Can you work these out from the model? Positions are in its coordinate system, mm. A direction names the side the tool comes from. Coordinates: 2 decimals unless noted, no trailing zeros. Order: outer loops, then holes, each group sorted by start corner. A loop starts at its lowest first (then second) coordinate and runs counter-clockwise, first axis right, second up.
Autodesk Inventor part; units mm, degrees
ref_plane "Work Plane1" through (220.5144, 586.5816, 98.3522) normal (0, 0, 1) x (1, 0, 0)
ref_plane "YZ Plane" through (0, 0, 0) normal (1, 0, 0) x (0, 1, 0)
ref_plane "XZ Plane" through (0, 0, 0) normal (0, 1, 0) x (-1, 0, 0)
ref_plane "Work Plane1" through (220.5144, 586.5816, 98.3522) normal (0, 0, 1) x (1, 0, 0)
sketch "Sketch1" plane through (220.5144, 586.5816, 98.3522) normal (0, 0, 1) x (1, 0, 0)
  line L0 (12.7, 622.3) -> (215.9, 622.3)
  line L1 (12.7, 317.5) -> (215.9, 317.5)
  line L2 (241.3, 317.5) -> (241.3, 596.9)
  line L3 (-12.7, 596.9) -> (-12.7, 317.5)
  line L4 (215.9, 596.9) -> (12.7, 596.9)
  line L5 (215.9, 596.9) -> (215.9, 317.5)
  line L6 (12.7, 317.5) -> (12.7, 596.9)
  line L7 (212.725, 593.725) -> (15.875, 593.725)
  line L8 (15.875, 593.725) -> (15.875, 320.675)
  line L9 (15.875, 320.675) -> (212.725, 320.675)
  line L10 (212.725, 320.675) -> (212.725, 593.725)
  point P0 (-220.5144, -586.5816)
extrude "Extrusion1" add sketch "Sketch1" along normal blind 127 and the other way blind 25.4 contours L10 L9 L8 L7
shell "Shell1" thickness 12.7 removed faces 1 at (302.006, 1089.2899, 225.3522)
sketch "Sketch2" plane through (433.2394, 907.2566, 225.3522) normal (1, 0, 0) x (0, 0, -1)
  line L0 (64.2794, 112.1381) -> (64.2794, 158.5332) construction
  line L1 (64.2794, 158.5332) -> (96.9042, 158.5332) construction
  line L2 (96.9042, 158.5332) -> (96.9042, 112.1381) construction
  line L3 (96.9042, 112.1381) -> (64.2794, 112.1381) construction
  line L4 (3.9697, 3.4317) -> (3.9697, 49.8268) construction
  line L5 (3.9697, 49.8268) -> (36.5945, 49.8268) construction
  line L6 (36.5945, 49.8268) -> (36.5945, 3.4317) construction
  line L7 (36.5945, 3.4317) -> (3.9697, 3.4317) construction
  point P0 (225.3522, -907.2566)
sketch "Sketch3" plane through (236.3894, 907.2566, 225.3522) normal (-1, 0, 0) x (0, 0, 1)
  line L0 (-63.2632, 158.0563) -> (-63.2632, 111.6612) construction
  line L1 (-63.2632, 111.6612) -> (-95.888, 111.6612) construction
  line L2 (-95.888, 111.6612) -> (-95.888, 158.0563) construction
  line L3 (-95.888, 158.0563) -> (-63.2632, 158.0563) construction
  line L4 (-5.0298, 267.8039) -> (-5.0298, 221.4088) construction
  line L5 (-5.0298, 221.4088) -> (-37.6546, 221.4088) construction
  line L6 (-37.6546, 221.4088) -> (-37.6546, 267.8039) construction
  line L7 (-37.6546, 267.8039) -> (-5.0298, 267.8039) construction
  point P0 (-225.3522, -907.2566)
properties part number "Bucket yellow"
1. Please list where these lines run through material, in increasing order: probe 1 along X at (y, z) = (951.5, 185); probe 2 along Y at (x, z) = (276, 88); probe 3 along Z at (x, y) = (379, 989.5).
Completed:
probe 1: x = 236.39 to 249.09, 420.54 to 433.24
probe 2: y = 907.26 to 919.96, 1167.61 to 1180.31
probe 3: z = 72.95 to 85.65
2. Thinking about a two-plate mould opening in X: for faces 1 (the flat face through (433.239, 1042, 148)), 2 (the flat face through (247, 1055, 225.352)), 3 (the flat face through (336, 1167.607, 155)), which applies, pulls with the +X half, pulls with the -X half, needs draft (parallel to the pull), parting line crosses it, or undercut?
Completed:
face 1: pulls with the +X half
face 2: needs draft
face 3: undercut
3. Imagine slicing it at B-B on y = 930.5. Please give me the cut outline in (x, z).
Completed:
outline: (236.39, 72.95) - (433.24, 72.95) - (433.24, 225.35) - (420.54, 225.35) - (420.54, 85.65) - (249.09, 85.65) - (249.09, 225.35) - (236.39, 225.35) - close
4. Imagine slicing it at C-C on x = 358. Please give me the cut outline in (y, z).
Completed:
outline: (907.26, 72.95) - (1180.31, 72.95) - (1180.31, 225.35) - (1167.61, 225.35) - (1167.61, 85.65) - (919.96, 85.65) - (919.96, 225.35) - (907.26, 225.35) - close
5. On a 3-axis mill with a long thin cutter (end or side, diameter ignored), from which of +Z, -Z, +X, -X, +Y, -Y can I reach the whole of each face in a straight line? I mean faces 4 (the flat face through (236.389, 1046, 148)), 5 (the flat face through (249.089, 1046, 155)). Say none if no direction works.
Completed:
face 4: +Z, -Z, -X, +Y, -Y
face 5: +Z
6. Imagine slicing it at A-A on z = 176.5. Please give me the cut outline in (x, y), then the cut area to 3 significant figures.
Completed:
outline: (236.39, 907.26) - (433.24, 907.26) - (433.24, 1180.31) - (236.39, 1180.31) - close; hole (249.09, 919.96) - (420.54, 919.96) - (420.54, 1167.61) - (249.09, 1167.61) - close
area: 11,300 mm2
